from build123d import *

# Parameters (mm, degrees)
SKETCH_1_W          = 240
SKETCH_1_H          = 65
SKETCH_1_R          = 2.1
EXTRUDE_1_DEPTH     = 3
FILLET_1_R          = 5
SKETCH_5_R          = 2.1
CUT_EXTRUDE_4_DEPTH = 10
SKETCH_3_R          = 6
SKETCH_3_R_2        = 2.05
CUT_EXTRUDE_5_DEPTH = 10


with BuildPart() as part:
    # 草图1 → 凸台-拉伸1 (new body)
    # profile 1 of 2: a face of its own
    with BuildSketch(Plane(origin=(0, 0, 0), x_dir=(1, 0, 0), z_dir=(0, 1, 0))):
        with Locations((0, 23.125)):
            Rectangle(SKETCH_1_W, SKETCH_1_H)
        with Locations(Location((105, 10.625, 0), (0, 0, 270))):
            Circle(SKETCH_1_R, mode=Mode.SUBTRACT)
        with Locations(Location((-105, 10.625, 0), (0, 0, 270))):
            Circle(SKETCH_1_R, mode=Mode.SUBTRACT)
        with Locations(Location((-105, 45.625, 0), (0, 0, 270))):
            Circle(SKETCH_1_R, mode=Mode.SUBTRACT)
        with Locations(Location((105, 45.625, 0), (0, 0, 270))):
            Circle(SKETCH_1_R, mode=Mode.SUBTRACT)
    # profile 2 of 2: a face of its own
    with BuildSketch(Plane(origin=(0, 0, 0), x_dir=(1, 0, 0), z_dir=(0, 1, 0))):
        Polygon((13.003862914, -9.375), (-55, -9.375), (-55, -134.375), (55, -134.375), (55, -9.375), align=None)
    extrude(amount=EXTRUDE_1_DEPTH)

    # 圆角1
    fillet_1_edges = [part.edges().sort_by_distance(p)[0] for p in [
        (-120, 1.5, 9.375),
        (-120, 1.5, -55.625),
        (120, 1.5, -55.625),
        (120, 1.5, 9.375),
    ]]
    fillet(fillet_1_edges, radius=FILLET_1_R)

    # 草图5 → 切除-拉伸4 (cut)
    with BuildSketch(Plane(origin=(0, 3, 0), x_dir=(1, 0, 0), z_dir=(0, 1, 0))):
        with Locations(Location((-47.5, -124.375, 0), (0, 0, 270))):
            Circle(SKETCH_5_R)
        with Locations(Location((47.5, -124.375, 0), (0, 0, 270))):
            Circle(SKETCH_5_R)
        with Locations(Location((47.5, -99.375, 0), (0, 0, 270))):
            Circle(SKETCH_5_R)
        with Locations(Location((-47.5, -99.375, 0), (0, 0, 270))):
            Circle(SKETCH_5_R)
    extrude(amount=-CUT_EXTRUDE_4_DEPTH, mode=Mode.SUBTRACT)

    # 草图3 → 切除-拉伸5 (cut)
    with BuildSketch(Plane(origin=(0, 3, 0), x_dir=(1, 0, 0), z_dir=(0, 1, 0))):
        with Locations(Location((0, 24.469725565, 0), (0, 0, 270))):
            Circle(SKETCH_3_R)
        with Locations(Location((0, 4.469725565, 0), (0, 0, 270))):
            Circle(SKETCH_3_R_2)
        with Locations(Location((-17.320508076, 34.469725565, 0), (0, 0, 270))):
            Circle(SKETCH_3_R_2)
        with Locations(Location((17.320508076, 34.469725565, 0), (0, 0, 270))):
            Circle(SKETCH_3_R_2)
    extrude(amount=-CUT_EXTRUDE_5_DEPTH, mode=Mode.SUBTRACT)


solid = part.part
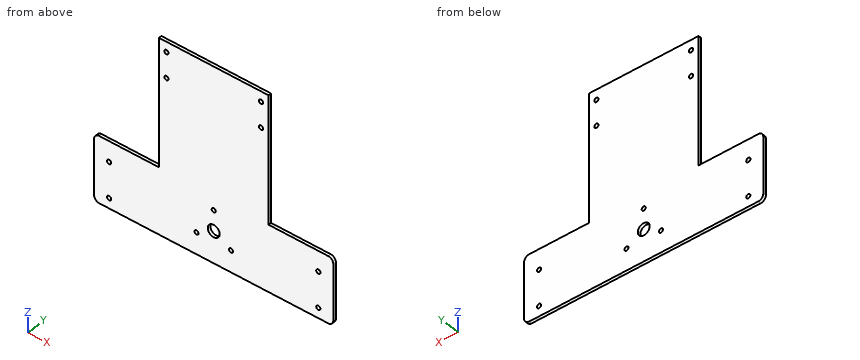
CAD build for the part. Positions are in the model's coordinates, mm. Give positions to 0.01 mm unless a question says otherwise; leave off trailing zeros. Loops run counter-clockwise (first coordinate to the right, second up) from the corner with the lowest first, then second, coordinate; pieces in that order, holes last. Notation, with made-up numbers: M 13,30.25 L 41,30.25 A30 cw 41,68.25 Z; hole C -20,61 d5. An arc over 180 degrees is marked long. One line per question, with ' | ' between items. Start each with the question number.
1. Flat gauge pins, fed straight in: pin 1 (0.9 mm diameter, centred on x = 73.5, y = 1.5, fed in from +Z) (3 decimals); pin 2 (0.9 mm diameter, centred on y = 2, z = 91, fed in from -X); pin 3 (1.5 mm diameter, centred on y = 0.5, z = 78, fed in from +X). Where does each tip first touch, or does it go through?
2. Saw through at A-A on y = 2.45. State how many separate pieces and enclosed holes the cut face has, plus the area to 3 significant figures.
3. Saw through at C-C on x = -71. Give the cut face in (y, z) (3 decimals), plus the area to 3 significant figures.
4. Probe L1, parallel to X at y = 2.35, z = -24; L2, parallel to X at y = 1.55, z = 13; L3, parallel to Z at x = 66, y = 1 (3 decimals). List the from-to ranges inside material, lowest first. Write a range as from..to.
5. Saw through at B-B on z = 16. Give the cut face in (x, y).
Result sheet:
1) pin 1: stops at z = 9.375 | pin 2: stops at x = -55 | pin 3: stops at x = 55
2) separate pieces: 1 | enclosed holes: 12 | area: 29,100 mm^2
3) outline: M 0,-55.625 L 3,-55.625 L 3,9.375 L 0,9.375 Z | area: 195 mm^2
4) L1: x = -120..-5.98, 5.98..120 | L2: x = -55..55 | L3: z = -55.625..9.375
5) outline: M -55,0 L 55,0 L 55,3 L -55,3 Z
